The model under review builds one solid part; all positions refer to its coordinate system, in mm. Face numbers are marked on the shaded views. A direction names the side the tool comes from. Round coordinates to 2 decimals unless told otherwise and drop trailing zeros. Loops run counter-clockwise (first coordinate to the right, second up) from the corner with the lowest first, then second, coordinate; pieces in that order, holes last. Notation, with made-up numbers: M -27,-31 L 7,-31 A23 cw 7,-7 Z; hole C -16.75,65 d11. An arc over 180 degrees is marked long. Answer as a JSON object with one key per item and string values. Group by question number.
Item 1: Consider section A-A (y = -43). Give the boundary of the cut face in (x, z).
Item 2: Consider section C-C (x = 100). Give the boundary of the cut face in (y, z), and give its area (3 significant figures).
Item 3: The part is to be moulded in two halves that separate along X. For the marked faces 1, 2 and 3, say which applies: +X half, -X half, draft (parallel to the pull), parting line (faces both ways), or undercut.
Item 4: Consider section D-D (z = -23). State how many separate pieces and enclosed holes the cut face has, and give its area (3 significant figures).
Item 5: Insertion check: P1, Ø22, axis at x = 108.5, y = -38, coming from the -Z side; P2, Ø21.5, axis at y = -21.5, z = -24, coming from the -X side; P3, Ø9, axis at x = -5.5, y = 11, coming from the +Z side; P4, Ø2.5, axis at x = 118, y = -39.5, coming from the -Z side. Each pin has a flat end and moves straight along its axis. Give the tip position at first contact, or say it passes through.
Item 6: Tool access review of the marked faces 4, 5 and 6: name each direction out of +Z, -Z, +X, -X, +Y, -Y from which nothing blocks a thin tool from reaching the whole face with its end or side.
Item 7: To check wall thickness, follow line 1 (X direction, y = -31, z = -23); line 2 (X direction, y = 9, z = -23); line 3 (X direction, y = -29, z = -23). State the ranges of each line that lie inside material, in increasing order.
Item 8: Consider section B-B (x = 26). Give the boundary of the cut face in (y, z), and give its area (3 significant figures).
```python
from build123d import *

# Parameters (mm, degrees)
SKETCH1_W           = 3
SKETCH1_H           = 40
BOSS_EXTRUDE1_DEPTH = 120
SKETCH9_W           = 120
SKETCH9_H           = 3
BOSS_EXTRUDE2_DEPTH = 40
SKETCH10_W          = 120
SKETCH10_H          = 40
SKETCH10_R          = 13.75
SKETCH10_R_2        = 7.6
SKETCH10_R_3        = 2.26
BOSS_EXTRUDE3_DEPTH = 2.3
SKETCH11_R          = 7
SKETCH11_R_2        = 2.25
SKETCH11_R_3        = 2.26
CUT_EXTRUDE5_DEPTH  = 4
SKETCH12_W          = 120
SKETCH12_H          = 43
SKETCH12_R          = 3.5
SKETCH12_R_2        = 12
SKETCH12_R_3        = 13.75
BOSS_EXTRUDE4_DEPTH = 3
SKETCH13_W          = 20
SKETCH13_H          = 20
SKETCH13_R          = 2.583718127
BOSS_EXTRUDE5_DEPTH = 5
BOSS_EXTRUDE6_DEPTH = 2
SKETCH15_W          = 15
SKETCH15_H          = 8
BOSS_EXTRUDE7_DEPTH = 3
SKETCH16_W          = 2
SKETCH16_H          = 8
BOSS_EXTRUDE8_DEPTH = 5


with BuildPart() as part:
    # Sketch1 → Boss-Extrude1 (new body)
    with BuildSketch(Plane(origin=(0, 0, 0), x_dir=(0, 0, -1), z_dir=(1, 0, 0))):
        with Locations((1.5, -13)):
            Rectangle(SKETCH1_W, SKETCH1_H)
    extrude(amount=BOSS_EXTRUDE1_DEPTH)

    # Sketch9 → Boss-Extrude2 (add)
    with BuildSketch(Plane(origin=(0, 0, -3), x_dir=(-1, 0, 0), z_dir=(0, 0, -1))):
        with Locations((-60, -31.5)):
            Rectangle(SKETCH9_W, SKETCH9_H)
    extrude(amount=BOSS_EXTRUDE2_DEPTH)

    # Sketch10 → Boss-Extrude3 (add)
    with BuildSketch(Plane(origin=(0, -30, 0), x_dir=(1, 0, 0), z_dir=(0, 1, 0))):
        with Locations((60, 23)):
            Rectangle(SKETCH10_W, SKETCH10_H)
        with Locations((100, 23)):
            Circle(SKETCH10_R, mode=Mode.SUBTRACT)
        with Locations((63, 23)):
            Circle(SKETCH10_R_2, mode=Mode.SUBTRACT)
        with Locations((26, 23)):
            Circle(SKETCH10_R_2, mode=Mode.SUBTRACT)
        with Locations((6, 23)):
            Circle(SKETCH10_R_3, mode=Mode.SUBTRACT)
    extrude(amount=BOSS_EXTRUDE3_DEPTH)

    # Sketch11 → Cut-Extrude5 (cut, through all)
    with BuildSketch(Plane(origin=(0, -30, 0), x_dir=(1, 0, 0), z_dir=(0, 1, 0))):
        with Locations((63, 23)):
            Circle(SKETCH11_R)
        with Locations((26, 23)):
            Circle(SKETCH11_R_2)
        with Locations((6, 23)):
            Circle(SKETCH11_R_3)
    extrude(amount=-CUT_EXTRUDE5_DEPTH, mode=Mode.SUBTRACT)

    # Sketch12 → Boss-Extrude4 (add)
    with BuildSketch(Plane(origin=(0, 7, 0), x_dir=(1, 0, 0), z_dir=(0, 1, 0))):
        with Locations((60, 21.5)):
            Rectangle(SKETCH12_W, SKETCH12_H)
        with Locations((6, 23)):
            Circle(SKETCH12_R, mode=Mode.SUBTRACT)
        with Locations((26, 23)):
            Circle(SKETCH12_R_2, mode=Mode.SUBTRACT)
        with Locations((63, 23)):
            Circle(SKETCH12_R_2, mode=Mode.SUBTRACT)
        with Locations((100, 23)):
            Circle(SKETCH12_R_3, mode=Mode.SUBTRACT)
    extrude(amount=BOSS_EXTRUDE4_DEPTH)

    # Sketch13 → Boss-Extrude5 (add)
    with BuildSketch(Plane(origin=(120, 0, 0), x_dir=(0, 0, -1), z_dir=(1, 0, 0))):
        with Locations((10, -43)):
            Rectangle(SKETCH13_W, SKETCH13_H)
        with Locations((10, -43)):
            Circle(SKETCH13_R, mode=Mode.SUBTRACT)
    extrude(amount=-BOSS_EXTRUDE5_DEPTH)

    # Sketch14 → Boss-Extrude6 (add)
    with BuildSketch(Plane.XY):
        Polygon((115, -53), (115, -33), (95, -33), align=None)
    extrude(amount=-BOSS_EXTRUDE6_DEPTH)

    # Sketch15 → Boss-Extrude7 (add)
    with BuildSketch(Plane(origin=(0, 10, 0), x_dir=(1, 0, 0), z_dir=(0, 1, 0))):
        with Locations((-7.5, 39)):
            Rectangle(SKETCH15_W, SKETCH15_H)
    extrude(amount=-BOSS_EXTRUDE7_DEPTH)

    # Sketch16 → Boss-Extrude8 (add)
    with BuildSketch(Plane(origin=(0, 10, 0), x_dir=(1, 0, 0), z_dir=(0, 1, 0))):
        with Locations((-14, 39)):
            Rectangle(SKETCH16_W, SKETCH16_H)
    extrude(amount=BOSS_EXTRUDE8_DEPTH)


solid = part.part
```
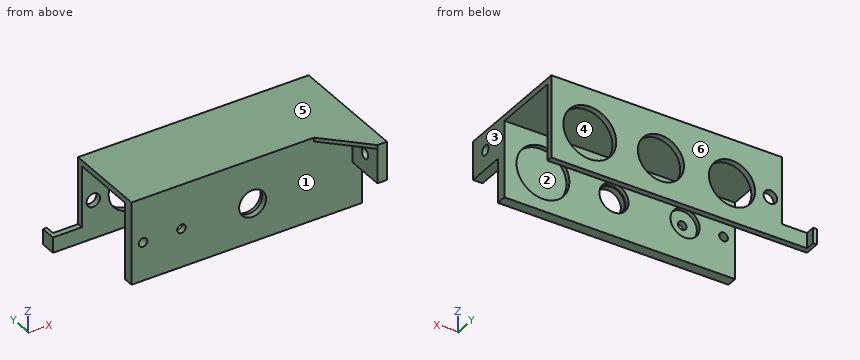
Geometry results:
{
 "1": {"outline": "M 105,-2 L 115,-2 L 115,-7.42 L 120,-7.42 L 120,0 L 105,0 Z; M 115,-20 L 120,-20 L 120,-12.58 L 115,-12.58 Z"},
 "2": {"outline": "M -38,-2 L -33,-2 L -33,-43 L -27.7,-43 L -27.7,-36.75 L -30,-36.75 L -30,-9.25 L -27.7,-9.25 L -27.7,-3 L 7,-3 L 7,-9.25 L 10,-9.25 L 10,0 L -38,0 Z; M 7,-43 L 10,-43 L 10,-36.75 L 7,-36.75 Z", "area": "325 mm^2"},
 "3": {"face 1": "draft", "face 2": "undercut", "face 3": "+X half"},
 "4": {"separate pieces": "9", "enclosed holes": "0", "area": "536 mm^2"},
 "5": {"P1": "stops at z = -43", "P2": "stops at x = 0", "P3": "stops at z = -35", "P4": "stops at z = -20"},
 "6": {"face 4": "-Z, +X, -X", "face 5": "+Z, +X, -X, +Y, -Y", "face 6": "+Z, -Z, +X, +Y"},
 "7": {"line 1": "x = 0 to 3.74, 8.26 to 23.75, 28.25 to 56, 70 to 120", "line 2": "x = 0 to 2.5, 9.5 to 14, 38 to 51, 75 to 86.25, 113.75 to 120", "line 3": "x = 0 to 3.74, 8.26 to 18.4, 33.6 to 55.4, 70.6 to 86.25, 113.75 to 120"},
 "8": {"outline": "M -33,-43 L -27.7,-43 L -27.7,-30.6 L -30,-30.6 L -30,-25.25 L -33,-25.25 Z; M -33,-20.75 L -30,-20.75 L -30,-15.4 L -27.7,-15.4 L -27.7,-3 L 7,-3 L 7,-11 L 10,-11 L 10,0 L -33,0 Z; M 7,-43 L 10,-43 L 10,-35 L 7,-35 Z", "area": "341 mm^2"}
}
